Verification items for the finished model (mm, model axes). Face numbers are marked on the shaded views. Coordinates: 2 decimals unless noted, no trailing zeros. Order: outer loops, then holes, each group sorted by start corner. A loop starts at its lowest first (then second) coordinate and runs counter-clockwise, first axis right, second up. Notation, with made-up numbers: (58.25, -8.5) -> (105.25, -8.5) arc R15 ccw to (105.25, 6.5) -> close; hole circle Ø9 at (54, -36). An arc over 180 degrees is marked (long way). Write item = value, one per line. Start each with the question number.
from build123d import *

# Parameters (mm, degrees)
SKETCH_1_W                  = 10
SKETCH_1_H                  = 6
REVOLVE_1_ANGLE             = 75
HOLE_WIZARD_M31_D           = 3.4
HOLE_WIZARD_M31_CBORE_D     = 6.05
HOLE_WIZARD_M31_CBORE_DEPTH = 3
FILLET_1_R                  = 2
FILLET_2_R                  = 3


with BuildPart() as part:
    # Эскиз1 → Повернуть1 (revolve)
    with BuildSketch(Plane(origin=(0, 0, 0), x_dir=(0, 1, 0), z_dir=(0.9659258262890689, 0, -0.258819045102519))):
        with Locations((5, -41.5)):
            Rectangle(SKETCH_1_W, SKETCH_1_H)
    revolve(axis=Axis((0, 10, 0), (0, 1, 0)), revolution_arc=REVOLVE_1_ANGLE)

    # Цековка для винта с заклепочной головкой M31 (through all)
    with Locations(Plane(origin=(0, 10, 0), x_dir=(1, 0, 0), z_dir=(0, 1, 0))):
        with Locations((-40.085921791, 10.740990372), (-20.75, 35.940054257)):
            CounterBoreHole(HOLE_WIZARD_M31_D / 2, HOLE_WIZARD_M31_CBORE_D / 2, HOLE_WIZARD_M31_CBORE_DEPTH)

    # Скругление1
    fillet_1_edges = [part.edges().sort_by_distance(p)[0] for p in [
        (-11.517447507, 5, -42.98369927),
        (-44.5, 5, 0),
    ]]
    fillet(fillet_1_edges, radius=FILLET_1_R)

    # Скругление2
    fillet_2_edges = [part.edges().sort_by_distance(p)[0] for p in [
        (-38.5, 5, 0),
        (-9.964533236, 5, -37.188144312),
    ]]
    fillet(fillet_2_edges, radius=FILLET_2_R)


solid = part.part
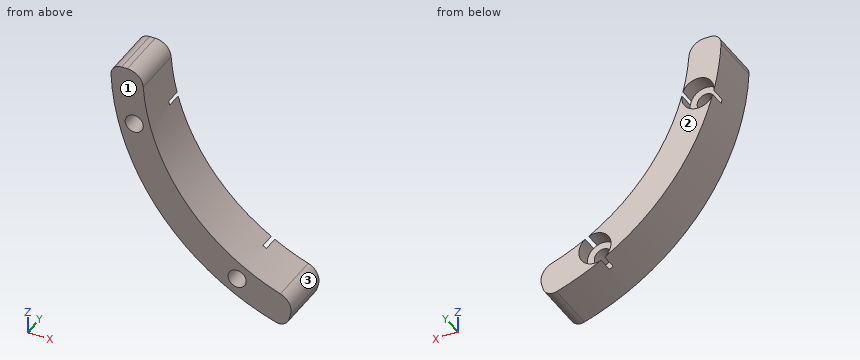
Item 1: Section check D-D (x = -28.5). Record the boundary of the cut face in (y, z).
Item 2: Section check B-B (y = 5). Record the boundary of the cut face in (x, z).
Item 3: Thickness scan on line 1 (Z direction, x = -20.75, y = 5.75); line 2 (X direction, y = 4, z = -11); line 3 (X direction, y = 8, z = -28.5). Record the ranges inside material, lowest first.
Item 4: Section check A-A (x = -20.75). Record the boundary of the cut face in (y, z), then the cut area to 3 significant figures.
Item 5: Section check C-C (y = 8). State how many separate pieces and enclosed holes the cut face has, then the cut area to 3 significant figures.
Item 6: Gauge pin test, flat ends, axial feed: P1, Ø2.5, axis at x = -20.75, z = -35.94, coming from the +Y side; P2, Ø3, axis at x = -39, z = -11.5, coming from the +Y side; P3, Ø2, axis at x = -40.5, y = 5.5, coming from the -Z side; P4, Ø3, axis at y = 3.5, z = -8.5, coming from the +X side. Record the tip position at first contact, or that the pin passes through.
Item 7: Mould release check, pull along Y, two halves, no side actions. Record for the marked faces 1, 2 and 3: pulls with the +Y half, pulls with the -Y half, needs draft (parallel to the pull), parting line crosses it, or undercut.
Filled sheet:
q1.outline = (0, -34.18) -> (10, -34.18) -> (10, -25.88) -> (0, -25.88) -> close
q2.outline = (-44.45, -2.09) arc R44.5 ccw to (-13.53, -42.39) arc R2 ccw to (-10.99, -41.01) -> (-10.71, -39.98) arc R3 ccw to (-12.63, -36.37) arc R38.5 cw to (-38.4, -2.78) arc R3 ccw to (-41.39, 0) -> (-42.45, 0) arc R2 ccw to start; hole circle Ø3.4 at (-40.09, -10.74); hole circle Ø3.4 at (-20.75, -35.94)
q3.line_1 = -39.37 to -37.64, -34.24 to -32.43
q3.line_2 = -43.12 to -41.77, -38.41 to -36.9
q3.line_3 = -34.18 to -25.88
q4.outline = (0, -39.37) -> (10, -39.37) -> (10, -38.97) -> (7, -38.97) -> (7, -37.64) -> (0, -37.64) -> close; (0, -34.24) -> (7, -34.24) -> (7, -32.92) -> (10, -32.92) -> (10, -32.43) -> (0, -32.43) -> close
q4.area = 27.4 mm^2
q5.separate_pieces = 3
q5.enclosed_holes = 0
q5.area = 263 mm^2
q6.P1 = through
q6.P2 = 7
q6.P3 = -20.49
q6.P4 = -37.18
q7.face_1 = pulls with the -Y half
q7.face_2 = pulls with the +Y half
q7.face_3 = needs draft
